```python
from build123d import *

# Parameters (mm, degrees)
SKETCH1_R           = 14.097
BOSS_EXTRUDE1_DEPTH = 12.7


with BuildPart() as part:
    # Sketch1 → Boss-Extrude1 (new body)
    with BuildSketch(Plane(origin=(0, 0, 0), x_dir=(1, 0, 0), z_dir=(0, 1, 0))):
        with Locations(Location((0, 0, 0), (0, 0, 270))):  # turned: the seam where the file's is
            Circle(SKETCH1_R)
    extrude(amount=BOSS_EXTRUDE1_DEPTH)

    # Sketch2 → Cut-Revolve1 (revolve, cut)
    with BuildSketch(Plane.XY, mode=Mode.PRIVATE) as cut_revolve1_sk:
        with BuildLine():
            Line((4.953, 12.7), (4.953, 11.938))
            Line((4.953, 11.938), (8.382, 11.938))
            Line((8.382, 11.938), (8.382, 9.652))
            Line((8.382, 9.652), (12.573, 7.232325022))
            ThreePointArc((12.573, 7.232325022), (13.130822715, 6.674502306), (13.335, 5.912502306))
            Line((13.335, 5.912502306), (13.335, 0))
            Line((13.335, 0), (0, 0))
            Line((0, 0), (0, 12.7))
            Line((0, 12.7), (4.953, 12.7))
        make_face()
    revolve(cut_revolve1_sk.sketch.rotate(Axis((0, 0, 0), (0, 1, 0)), 90), axis=Axis((0, 0, 0), (0, 1, 0)), mode=Mode.SUBTRACT)  # turned: the seam where the file's is

    # Sketch3 → Cut-Revolve2 (revolve, cut)
    with BuildSketch(Plane.XY, mode=Mode.PRIVATE) as cut_revolve2_sk:
        with BuildLine():
            Line((14.097, 12.7), (14.097, 7.62))
            Line((14.097, 7.62), (9.906, 10.039674978))
            ThreePointArc((9.906, 10.039674978), (9.348177285, 10.597497694), (9.144, 11.359497694))
            Line((9.144, 11.359497694), (9.144, 12.7))
            Line((9.144, 12.7), (14.097, 12.7))
        make_face()
    revolve(cut_revolve2_sk.sketch.rotate(Axis((0, 0, 0), (0, 1, 0)), 90), axis=Axis((0, 0, 0), (0, 1, 0)), mode=Mode.SUBTRACT)  # turned: the seam where the file's is


solid = part.part
```
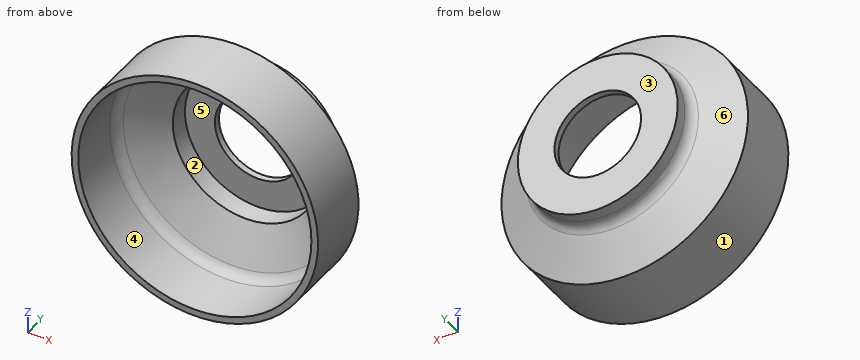
Model file for the job. Use its own axes, mm. Face numbers are marked on the shaded views. A direction names the side the tool comes from. Round coordinates to 2 decimals unless told otherwise and drop trailing zeros. Write each loop counter-clockwise with the first axis right and the second up, starting at its lowest first coordinate (ties: lowest second). Pieces come first, ordered by that corner, then holes. Notation, with made-up numbers: (-7.75, 57) - (-3.75, 57) arc R24 cw to (-3.75, 75) - close; hole circle Ø3 at (53, 62.5). An arc over 180 degrees is marked (long way). Use CSV: the item, a comma, the result in double quotes. Start each with the question number.
Item 1: Pin check, flat tips, straight feed: P1, Ø3, axis at y = 3.5, z = 6.5, coming from the -X side; P2, Ø3, axis at x = -11, z = -6.5, coming from the +Y side; P3, Ø5, axis at x = 0, z = -3.5, coming from the -Y side. Stop position of each tip, or through.
Item 2: Tool access for the marked faces 1 and 2: list every direction of +Z, -Z, +X, -X, +Y, -Y with a clear straight run to the whole face (end or side of a thin tool).
Item 3: Band-saw the part on C-C (y = 1). Write the cut outline in (x, z) (3 decimals), and give its area (3 significant figures).
Item 4: Band-saw the part on B-B (x = 0). Write the cut outline in (y, z) (1 decimal), and give its area (3 significant figures).
Item 5: Band-saw the part on A-A (z = 0). Write the cut outline in (x, y) (1 decimal).
Item 6: Two-plate mould, pull along X, no slides. Class the marked faces 3, 4, 5 and 6: released by +X, released by -X, zero draft, split by the parting line, or undercut.
Item 7: Drill centre lines: L1, parallel to X at y = 1.45, z = 0 (3 decimals); L2, parallel to X at y = 12.2, z = 0; L3, parallel to Z at x = -9.75, y = 3.25. Where is each one in solid material? Low to high. Write a range as [from, to].
Checked values:
1,P1,"stops at x = -13.18"
1,P2,"stops at y = 9.25"
1,P3,"stops at y = 11.94"
2,face 1,"+Y, -Y"
2,face 2,"-Y"
3,outline,"circle Ø28.194 at (0, 0); hole circle Ø26.67 at (0, 0)"
3,area,"65.7 mm²"
4,outline,"(0, -14.1) - (7.6, -14.1) - (10, -9.9) arc R1.5 cw to (11.4, -9.1) - (12.7, -9.1) - (12.7, -5) - (11.9, -5) - (11.9, -8.4) - (9.7, -8.4) - (7.2, -12.6) arc R1.5 cw to (5.9, -13.3) - (0, -13.3) - close; (0, 13.3) - (5.9, 13.3) arc R1.5 cw to (7.2, 12.6) - (9.7, 8.4) - (11.9, 8.4) - (11.9, 5) - (12.7, 5) - (12.7, 9.1) - (11.4, 9.1) arc R1.5 cw to (10, 9.9) - (7.6, 14.1) - (0, 14.1) - close"
4,area,"33.3 mm²"
5,outline,"(-14.1, 0) - (-13.3, 0) - (-13.3, 5.9) arc R1.5 cw to (-12.6, 7.2) - (-8.4, 9.7) - (-8.4, 11.9) - (-5, 11.9) - (-5, 12.7) - (-9.1, 12.7) - (-9.1, 11.4) arc R1.5 cw to (-9.9, 10) - (-14.1, 7.6) - close; (5, 11.9) - (8.4, 11.9) - (8.4, 9.7) - (12.6, 7.2) arc R1.5 cw to (13.3, 5.9) - (13.3, 0) - (14.1, 0) - (14.1, 7.6) - (9.9, 10) arc R1.5 cw to (9.1, 11.4) - (9.1, 12.7) - (5, 12.7) - close"
6,face 3,"zero draft"
6,face 4,"undercut"
6,face 5,"undercut"
6,face 6,"split by the parting line"
7,L1,"x = [-14.097, -13.335], [13.335, 14.097]"
7,L2,"x = [-9.14, -4.95], [4.95, 9.14]"
7,L3,"z = [-10.18, -9.1], [9.1, 10.18]"
